For this review, take the finished solid that the model builds, in its own axes (mm). Give positions to 0.01 mm unless a question says otherwise; leave off trailing zeros. Write each loop counter-clockwise with the first axis right and the second up, starting at its lowest first coordinate (ties: lowest second). Pieces come first, ordered by that corner, then holes. Notation, with made-up numbers: M 18.5,8.5 L 29.5,8.5 A33 ccw 29.5,38.5 Z; hole C -21,46.25 d5. An arc over 180 degrees is marked long. Use one line per item in the form item = value. Start each with the question number.
Q1. Consider section C-C on z = -6. Write out the cut boundary in (x, y), and give its area (3 significant figures).
Q2. Consider section D-D on y = -7. Give the number of separate pieces and of enclosed holes in the cut face, and give its area (3 significant figures).
Q3. For probe 1 along X at (y, z) = (9, 0); probe 2 along X at (y, z) = (0, 16); probe 3 along X at (y, z) = (0, 17), list the stretches that pass through material, from the lowest coordinate up. Write a range as [from, to].
Q4. Consider section A-A on z = 0. Write out the cut boundary in (x, y).
Q5. Consider section B-B on y = 13. Write out the cut boundary in (x, z).
Q6. Mouldability with a two-part tool opening along Y and no side actions: class faces 1 (the flat face through (1, 19, 0)), 2 (the flat face through (1, -19, 0)), 3 (the cylindrical face through (37.53, -0.27, 1.61)), 4 (the cylindrical face through (10.74, 2.38, 16.81)) as released by +Y, released by -Y, zero draft, split by the parting line, or undercut.
```python
from build123d import *

# Parameters (mm, degrees)
SKETCH1_R           = 3
BOSS_EXTRUDE1_DEPTH = 19


with BuildPart() as part:
    # Sketch1 → Boss-Extrude1 (new, symmetric)
    with BuildSketch(Plane(origin=(0, 0, 0), x_dir=(1, 0, 0), z_dir=(0, 1, 0))):
        with BuildLine():
            Line((-35, 19), (35, 19))
            ThreePointArc((35, 19), (54, 0), (35, -19))
            Line((35, -19), (-35, -19))
            ThreePointArc((-35, -19), (-54, 0), (-35, 19))
        make_face()
        with Locations(Location((-35, 0, 0), (0, 0, 270))):
            Circle(SKETCH1_R, mode=Mode.SUBTRACT)
        with Locations(Location((35, 0, 0), (0, 0, 270))):
            Circle(SKETCH1_R, mode=Mode.SUBTRACT)
    extrude(amount=BOSS_EXTRUDE1_DEPTH, both=True)

    # Sketch3 → M24x2.0 Tapped Hole1 (revolve, cut)
    with BuildSketch(Plane(origin=(0, 0, 19), x_dir=(0, -1, 0), z_dir=(1, 0, 0))):
        Polygon((0, 0), (0, 10), (11, 3.390533191), (11, 1.025), (12.025, 0), align=None)
    revolve(axis=Axis((0, 0, 25.35), (0, 0, -1)), mode=Mode.SUBTRACT)


solid = part.part
```
Working result:
q1.outline = M -53.03,-19 L 53.03,-19 L 53.03,19 L -53.03,19 Z
q1.area = 4,030 mm²
q2.separate_pieces = 1
q2.enclosed_holes = 2
q2.area = 3,650 mm²
q3.probe_1 = [-54, -38], [-32, 32], [38, 54]
q3.probe_2 = [-45.25, -11], [11, 45.25]
q3.probe_3 = [-43.49, -11], [11, 43.49]
q4.outline = M -54,-19 L -38,-19 L -38,19 L -54,19 Z; M -32,-19 L 32,-19 L 32,19 L -32,19 Z; M 38,-19 L 54,-19 L 54,19 L 38,19 Z
q5.outline = M -35,-19 L 35,-19 A19 ccw 35,19 L -35,19 A19 ccw Z; hole C -35,0 d6; hole C 35,0 d6
q6.face_1 = released by +Y
q6.face_2 = released by -Y
q6.face_3 = zero draft
q6.face_4 = undercut
